Source: CAD feature listing. Evaluate the final solid. Frame: model axes, mm. Round coordinates to 2 decimals unless told otherwise and drop trailing zeros. Loops run counter-clockwise (first coordinate to the right, second up) from the corner with the lowest first, then second, coordinate; pieces in that order, holes last. Notation, with made-up numbers: M -30.5,-29.5 L 1.5,-29.5 A9 ccw 1.5,-14.5 Z; hole C 29,68 d1. An arc over 180 degrees is marked long. Write each question's results on one line, items separated by ' | '. Start each with the question number.
1. Section C-C on x = 107. Output: boundary loops of the cut face in (y, z), and give its area (3 significant figures).
2. Ray query, line 1 (Y direction, x = 0, z = 8.25); line 2 (X direction, y = -1.5, z = 5.5); line 3 (Y direction, x = -46, z = 8). Return the intervals inside material, ascending.
3. Contact query for flat-ended pins moving along their axis: pin 1 Ø8 at (x, y) = (60.62, 35) entering from +Z; pin 2 Ø2 at (y, z) = (-67.5, 3) entering from -X; pin 3 Ø1 at (x, z) = (20.5, 1) entering from -Y; pin 4 Ø1 at (y, z) = (-36.5, 8) entering from +X. Output: stop coordinate, or through.
4. Section B-B on z = 3.75. Give the number of separate pieces and of enclosed holes in the cut face, and give its area (3 significant figures).
5. Section A-A on y = 28. Output: boundary loops of the cut face in (x, z), and give its area (3 significant figures).
6. Section D-D on y = -81.5. Output: boundary loops of the cut face in (x, z), and give its area (3 significant figures).
from build123d import *

# Parameters (mm, degrees)
SKETCH_1_R          = 130
SKETCH_1_R_2        = 60
EXTRUDE_1_DEPTH     = 10
SKETCH_2_R          = 2.5
CUT_EXTRUDE_1_DEPTH = 185.119526395
SKETCH_3_R          = 2.5
CUT_EXTRUDE_2_DEPTH = 185.119526395


with BuildPart() as part:
    # 草图1 → 凸台-拉伸1 (new body)
    with BuildSketch(Plane.XY):
        Circle(SKETCH_1_R)
        Circle(SKETCH_1_R_2, mode=Mode.SUBTRACT)
    extrude(amount=EXTRUDE_1_DEPTH)

    # 草图2 → 切除-拉伸1 (cut, through all)
    with BuildSketch(Plane.XY.offset(10)):
        with Locations((0, 70)):
            Circle(SKETCH_2_R)
        with Locations((60.621778265, 35)):
            Circle(SKETCH_2_R)
        with Locations((60.621778265, -35)):
            Circle(SKETCH_2_R)
        with Locations((0, -70)):
            Circle(SKETCH_2_R)
        with Locations((-60.621778265, -35)):
            Circle(SKETCH_2_R)
        with Locations((-60.621778265, 35)):
            Circle(SKETCH_2_R)
    extrude(amount=-CUT_EXTRUDE_1_DEPTH, mode=Mode.SUBTRACT)

    # 草图3 → 切除-拉伸2 (cut, through all)
    with BuildSketch(Plane.XY.offset(10)):
        with Locations((0, 115)):
            Circle(SKETCH_3_R)
        with Locations((57.5, 99.592921435)):
            Circle(SKETCH_3_R)
        with Locations((99.592921435, 57.5)):
            Circle(SKETCH_3_R)
        with Locations((115, 0)):
            Circle(SKETCH_3_R)
        with Locations((99.592921435, -57.5)):
            Circle(SKETCH_3_R)
        with Locations((57.5, -99.592921435)):
            Circle(SKETCH_3_R)
        with Locations((0, -115)):
            Circle(SKETCH_3_R)
        with Locations((-57.5, -99.592921435)):
            Circle(SKETCH_3_R)
        with Locations((-99.592921435, -57.5)):
            Circle(SKETCH_3_R)
        with Locations((-115, 0)):
            Circle(SKETCH_3_R)
        with Locations((-99.592921435, 57.5)):
            Circle(SKETCH_3_R)
        with Locations((-57.5, 99.592921435)):
            Circle(SKETCH_3_R)
    extrude(amount=-CUT_EXTRUDE_2_DEPTH, mode=Mode.SUBTRACT)


solid = part.part
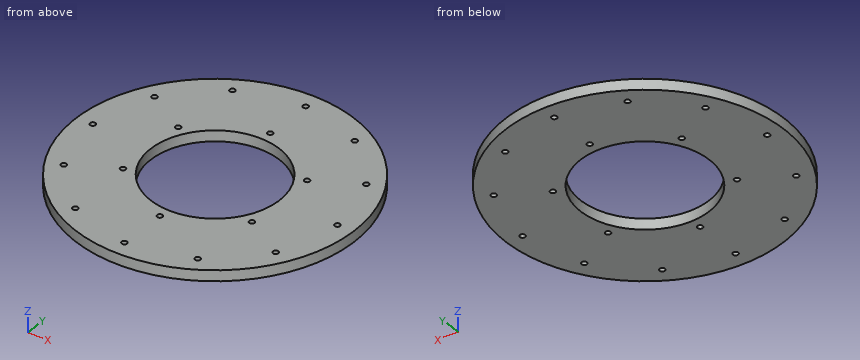
Taken from the geometry:
1) outline: M -73.83,0 L 73.83,0 L 73.83,10 L -73.83,10 Z | area: 1,480 mm^2
2) line 1: -130 to -117.5, -112.5 to -72.5, -67.5 to -60, 60 to 67.5, 72.5 to 112.5, 117.5 to 130 | line 2: -129.99 to -117, -113 to -59.98, 59.98 to 113, 117 to 129.99 | line 3: -121.59 to -38.52, 38.52 to 121.59
3) pin 1: z = 10 | pin 2: x = -111.7 | pin 3: y = -128.45 | pin 4: x = 124.92
4) separate pieces: 1 | enclosed holes: 19 | area: 41,400 mm^2
5) outline: M -126.95,0 L -53.07,0 L -53.07,10 L -126.95,10 Z; M 53.07,0 L 126.95,0 L 126.95,10 L 53.07,10 Z | area: 1,480 mm^2
6) outline: M -101.28,0 L 101.28,0 L 101.28,10 L -101.28,10 Z | area: 2,030 mm^2
